Geometry check sheet. Reference: the model listing, model coordinates, mm. A direction names the side the tool comes from. Round coordinates to 2 decimals unless told otherwise and drop trailing zeros. Write each loop counter-clockwise with the first axis right and the second up, starting at its lowest first coordinate (ties: lowest second). Pieces come first, ordered by that corner, then holes. Notation, with made-up numbers: M 25,-29.5 L 75,-29.5 A22 cw 75,4.5 Z; hole C 32.25,65 d2. An arc over 180 degrees is marked long. Use a Markdown table: item, result.
```python
from build123d import *

# Parameters (mm, degrees)
BOSS_EXTRUDE1_DEPTH = 6.35
CUT_EXTRUDE1_REACH  = 13.833
SKETCH2_R           = 1.75
FILLET1_R           = 0.2


with BuildPart() as part:
    # Sketch1 → Boss-Extrude1 (new body)
    with BuildSketch(Plane.XY):
        with BuildLine():
            Line((-11.5951, -3.038456882), (-11.5951, 3.038456882))
            Line((-11.5951, 3.038456882), (-11.539212407, 3.038456882))
            ThreePointArc((-11.539212407, 3.038456882), (-10.656027264, 3.404284146), (-10.2902, 4.287469289))
            Line((-10.2902, 4.287469289), (-10.2902, 6.402089023))
            ThreePointArc((-10.2902, 6.402089023), (-9.779862704, 7.166335846), (-8.878390822, 6.987825881))
            Line((-8.878390822, 6.987825881), (-5.582265308, 3.69923341))
            ThreePointArc((-5.582265308, 3.69923341), (-4.935610063, 2.733240723), (-4.7085, 1.593185507))
            Line((-4.7085, 1.593185507), (-4.7085, -1.593185507))
            ThreePointArc((-4.7085, -1.593185507), (-4.935610063, -2.733240723), (-5.582265308, -3.69923341))
            Line((-5.582265308, -3.69923341), (-8.878390822, -6.987825881))
            ThreePointArc((-8.878390822, -6.987825881), (-9.779862704, -7.166335846), (-10.2902, -6.402089023))
            Line((-10.2902, -6.402089023), (-10.2902, -4.287469289))
            ThreePointArc((-10.2902, -4.287469289), (-10.656027264, -3.404284146), (-11.539212407, -3.038456882))
            Line((-11.539212407, -3.038456882), (-11.5951, -3.038456882))
        make_face()
    extrude(amount=BOSS_EXTRUDE1_DEPTH)

    # Sketch2 → Cut-Extrude1 (cut, up to next)
    with BuildSketch(Plane.ZY.offset(11.5951), mode=Mode.PRIVATE) as cut_extrude1_sk1:
        with Locations((3.175, 0)):
            Circle(SKETCH2_R)
    cut_extrude1_tool1 = extrude(cut_extrude1_sk1.sketch, amount=-CUT_EXTRUDE1_REACH, mode=Mode.PRIVATE) & part.part
    add(cut_extrude1_tool1.solids().sort_by_distance((-11.5951, 0, 3.175))[0], mode=Mode.SUBTRACT)

    # Fillet1
    fillet1_edges = [part.edges().sort_by_distance(p)[0] for p in [
        (-11.5951, 0, 1.425),
    ]]
    fillet(fillet1_edges, radius=FILLET1_R)


solid = part.part
```
Item 1: Material ranges on line 1 along Z through (x, y) = (-9.75, 0) (3 decimals); line 2 along Y through (x, z) = (-6.75, 3.5); line 3 along Y through (x, z) = (-7, 3.75), recorded low to high. Write a range as from..to.
Outcome:
| item | result |
|---|---|
| line 1 | z = 0..1.425, 4.925..6.35 |
| line 2 | y = -4.86..-1.72, 1.72..4.86 |
| line 3 | y = -5.11..-1.65, 1.65..5.11 |
Item 2: Access from +Z, -Z, +X, -X, +Y, -Y to the whole of each face (thin tool, end or side, straight path). Record for faces 1 (the face through (-10.29, 5, 3)), 2 (the face through (-4.708, 0, 5.4)).
Outcome:
| item | result |
|---|---|
| face 1 | +Z, -Z, -X, +Y |
| face 2 | +Z, -Z, +X, +Y, -Y |
Item 3: Go/stop test with a flat-tipped pin: pin 1 (0.6 mm diameter, centred on y = -5.5, z = 4.5, fed in from -X). Record where the tip stops, or that it passes through.
Outcome:
| item | result |
|---|---|
| pin 1 | stops at x = -10.29 |
Item 4: Cross-section at D-D, the plane y = 6. Record the cut outline in (x, z).
Outcome:
| item | result |
|---|---|
| outline | M -10.29,0 L -7.89,0 L -7.89,6.35 L -10.29,6.35 Z |
Item 5: Cross-section at C-C, the plane x = -9.75. Record the cut outline in (y, z) (3 decimals).
Outcome:
| item | result |
|---|---|
| outline | M -7.178,0 L 7.178,0 L 7.178,6.35 L -7.178,6.35 Z; hole C 0,3.175 d3.5 |
Item 6: Mould release check, pull along Y, two halves, no side actions. Record for faces 3 (the face through (-10.29, -5, 3)), 4 (the face through (-4.93, -2.72, 3.13)), 5 (the face through (-8.1, -0.67, 4.79)): +Y half, -Y half, draft (parallel to the pull), parting line (faces both ways), or undercut.
Outcome:
| item | result |
|---|---|
| face 3 | draft |
| face 4 | -Y half |
| face 5 | undercut |
